Could you check a few things on this model? Use its own coordinates, in mm. A direction names the side the tool comes from. Give positions to 0.01 mm unless a question says otherwise; leave off trailing zeros. Write each loop counter-clockwise with the first axis right and the second up, starting at its lowest first coordinate (ties: lowest second). Pieces come first, ordered by that corner, then holes. Notation, with made-up numbers: (-38, 29.25) - (-2, 29.25) arc R28 ccw to (-2, 53.25) - close; hole circle Ø9 at (-33, -39.5). An arc over 180 degrees is marked (long way). Answer as CSV lines item,"result". Start each with the question number.
Q1. Imagine slicing it at D-D on x = 32. List the corners of the cut face in (y, z) for me.
Q2. Imagine slicing it at B-B on y = -10. List the corners of the cut face in (x, z) for me, and give its area (4 significant figures).
Q3. Will these pins go through, and if not, where does the flat tip stop? pin 1 Ø1.5 at (x, z) = (47, 1.5) entering from -Y; pin 2 Ø8 at (x, y) = (10, -95) entering from -Z; pin 3 Ø1 at (x, y) = (114.5, -31) entering from -Z; pin 4 Ø1.5 at (y, z) = (-57, 1.5) entering from -X.
Q4. If I drill on line 1 along Y through (x, z) = (10, 1.15); line 2 along X through (y, z) = (-93, 7); line 3 along Y through (x, z) = (81.5, 8.25), over which ranges is the centre line in solid material (lowest first)?
Q5. Imagine slicing it at A-A on z = 3.25. List the corners of the cut face in (x, y) for me, and give its area (3 significant figures).
Q6. Imagine slicing it at C-C on x = 85. List the corners of the cut face in (y, z) for me.
Q7. We'd pull the mould along Y, two halves only. Please class faces 3 (the face through (10.65, -97.93, 2.46)), 4 (the face through (102, -51, 5)): pulls with the +Y half, pulls with the -Y half, needs draft (parallel to the pull), parting line crosses it, or undercut.
Q8. On a 3-axis mill with a long thin cutter (end or side, diameter ignored), from which of +Z, -Z, +X, -X, +Y, -Y can I reach the whole of each face in a straight line? I mean faces 1 (the face through (46, -51, 10)), 2 (the face through (10.59, -90.54, 7.46)). Say none if no direction works.
```python
from build123d import *

# Parameters (mm, degrees)
SKETCH_1_W          = 95
SKETCH_1_H          = 105
EXTRUDE_3_DEPTH     = 10
SKETCH_10_R         = 4.5
CUT_EXTRUDE_4_DEPTH = 5
EXTRUDE_4_DEPTH     = 5
SKETCH_13_W         = 238
SKETCH_13_H         = 278
SKETCH_13_W_2       = 228
SKETCH_13_H_2       = 268
EXTRUDE_5_DEPTH     = 30
SKETCH_14_W         = 238
SKETCH_14_H         = 278
SKETCH_14_W_2       = 228
SKETCH_14_H_2       = 268
EXTRUDE_6_DEPTH     = 5
SKETCH_17_W         = 464.866912847
SKETCH_17_H         = 477.250662574
CUT_EXTRUDE_5_DEPTH = 30
SKETCH_10_2_R       = 4.5
CUT_EXTRUDE_6_DEPTH = 10
SKETCH_19_R         = 4.5
SKETCH_19_R_2       = 3
EXTRUDE_7_DEPTH     = 5


with BuildPart() as part:
    # Sketch 1 → Extrude 3 (new body)
    with BuildSketch(Plane.XY):
        with Locations((47.5, -52.5)):
            Rectangle(SKETCH_1_W, SKETCH_1_H)
    extrude(amount=EXTRUDE_3_DEPTH)

    # Sketch 10 → Cut-Extrude 4 (cut)
    with BuildSketch(Plane(origin=(0, 0, 0), x_dir=(-1, 0, 0), z_dir=(0, 0, -1))):
        with Locations((-85, -10)):
            Circle(SKETCH_10_R)
        with Locations((-85, -95)):
            Circle(SKETCH_10_R)
        with Locations((-10, -95)):
            Circle(SKETCH_10_R)
        with Locations((-10, -10)):
            Circle(SKETCH_10_R)
    extrude(amount=-CUT_EXTRUDE_4_DEPTH, mode=Mode.SUBTRACT)

    # Sketch 12 → Extrude 4 (add)
    with BuildSketch(Plane.XY.offset(10)):
        Polygon((47.5, 81.5), (161.5, 81.5), (161.5, -186.5), (-66.5, -186.5), (-66.5, 81.5), align=None)
    extrude(amount=-EXTRUDE_4_DEPTH)



with BuildPart() as body_2:
    # Sketch 13 → Extrude 5 (new body)
    with BuildSketch(Plane.XY.offset(10)):
        with Locations((47.5, -52.5)):
            Rectangle(SKETCH_13_W, SKETCH_13_H)
        with Locations((47.5, -52.5)):
            Rectangle(SKETCH_13_W_2, SKETCH_13_H_2, mode=Mode.SUBTRACT)
    extrude(amount=EXTRUDE_5_DEPTH)


with BuildPart() as part_1:
    add(part.part)

    add(body_2.part)  # Extrude 6 merges body 2
    # Sketch 14 → Extrude 6 (add)
    with BuildSketch(Plane(origin=(0, 0, 5), x_dir=(-1, 0, 0), z_dir=(0, 0, -1))):
        with Locations((-47.5, -52.5)):
            Rectangle(SKETCH_14_W, SKETCH_14_H)
        with Locations((-47.5, -52.5)):
            Rectangle(SKETCH_14_W_2, SKETCH_14_H_2, mode=Mode.SUBTRACT)
    extrude(amount=-EXTRUDE_6_DEPTH)

    # Sketch 17 → Cut-Extrude 5 (cut)
    with BuildSketch(Plane.XY.offset(40)):
        with Locations((32.258461874, -38.211058007)):
            Rectangle(SKETCH_17_W, SKETCH_17_H)
    extrude(amount=-CUT_EXTRUDE_5_DEPTH, mode=Mode.SUBTRACT)

    # Sketch 10_2 → Cut-Extrude 6 (cut)
    with BuildSketch(Plane(origin=(0, 0, 0), x_dir=(-1, 0, 0), z_dir=(0, 0, -1))):
        with Locations((-85, -10)):
            Circle(SKETCH_10_2_R)
        with Locations((-85, -95)):
            Circle(SKETCH_10_2_R)
        with Locations((-10, -95)):
            Circle(SKETCH_10_2_R)
        with Locations((-10, -10)):
            Circle(SKETCH_10_2_R)
    extrude(amount=-CUT_EXTRUDE_6_DEPTH, mode=Mode.SUBTRACT)

    # Sketch 19 → Extrude 7 (add)
    # profile 1 of 4: a face of its own
    with BuildSketch(Plane(origin=(0, 0, 0), x_dir=(-1, 0, 0), z_dir=(0, 0, -1))):
        with Locations((-85, -10)):
            Circle(SKETCH_19_R)
        with Locations((-85, -10)):
            Circle(SKETCH_19_R_2, mode=Mode.SUBTRACT)
    # profile 2 of 4: a face of its own
    with BuildSketch(Plane(origin=(0, 0, 0), x_dir=(-1, 0, 0), z_dir=(0, 0, -1))):
        with Locations((-10, -10)):
            Circle(SKETCH_19_R)
        with Locations((-10, -10)):
            Circle(SKETCH_19_R_2, mode=Mode.SUBTRACT)
    # profile 3 of 4: a face of its own
    with BuildSketch(Plane(origin=(0, 0, 0), x_dir=(-1, 0, 0), z_dir=(0, 0, -1))):
        with Locations((-85, -95)):
            Circle(SKETCH_19_R)
        with Locations((-85, -95)):
            Circle(SKETCH_19_R_2, mode=Mode.SUBTRACT)
    # profile 4 of 4: a face of its own
    with BuildSketch(Plane(origin=(0, 0, 0), x_dir=(-1, 0, 0), z_dir=(0, 0, -1))):
        with Locations((-10, -95)):
            Circle(SKETCH_19_R)
        with Locations((-10, -95)):
            Circle(SKETCH_19_R_2, mode=Mode.SUBTRACT)
    extrude(amount=-EXTRUDE_7_DEPTH)


solid = part_1.part
```
Conclusion:
1,outline,"(-191.5, 5) - (-105, 5) - (-105, 0) - (0, 0) - (0, 5) - (86.5, 5) - (86.5, 10) - (-191.5, 10) - close"
2,outline,"(-71.5, 5) - (0, 5) - (0, 0) - (7, 0) - (7, 5) - (5.5, 5) - (5.5, 10) - (-71.5, 10) - close; (13, 0) - (82, 0) - (82, 5) - (80.5, 5) - (80.5, 10) - (14.5, 10) - (14.5, 5) - (13, 5) - close; (88, 0) - (95, 0) - (95, 5) - (166.5, 5) - (166.5, 10) - (89.5, 10) - (89.5, 5) - (88, 5) - close"
2,area,"1,515 mm^2"
3,pin 1,"y = -105"
3,pin 2,"z = 0"
3,pin 3,"z = 5"
3,pin 4,"x = 0"
4,line 1,"-105 to -98, -92 to -13, -7 to 0"
4,line 2,"-71.5 to 5.97, 14.03 to 80.97, 89.03 to 166.5"
4,line 3,"-191.5 to -97.83, -92.17 to -12.83, -7.17 to 86.5"
5,outline,"(0, -105) - (95, -105) - (95, 0) - (0, 0) - close; hole circle Ø6 at (10, -95); hole circle Ø6 at (10, -10); hole circle Ø6 at (85, -95); hole circle Ø6 at (85, -10)"
5,area,"9,860 mm^2"
6,outline,"(-191.5, 5) - (-105, 5) - (-105, 0) - (-98, 0) - (-98, 5) - (-99.5, 5) - (-99.5, 10) - (-191.5, 10) - close; (-92, 0) - (-13, 0) - (-13, 5) - (-14.5, 5) - (-14.5, 10) - (-90.5, 10) - (-90.5, 5) - (-92, 5) - close; (-7, 0) - (0, 0) - (0, 5) - (86.5, 5) - (86.5, 10) - (-5.5, 10) - (-5.5, 5) - (-7, 5) - close"
7,face 3,"undercut"
7,face 4,"needs draft"
8,face 1,"+Z, +X, -X, +Y, -Y"
8,face 2,"+Z"
